```python
from build123d import *

# Parameters (mm, degrees)
SKETCH1_W           = 410
SKETCH1_H           = 70
BOSS_EXTRUDE1_DEPTH = 6
SKETCH2_W           = 6
SKETCH2_H           = 70
BOSS_EXTRUDE2_DEPTH = 25
SKETCH3_R           = 2.5
CUT_EXTRUDE1_DEPTH  = 418.891673384
SKETCH4_W           = 70
SKETCH4_H           = 8
CUT_EXTRUDE2_DEPTH  = 418.891673384


with BuildPart() as part:
    # Sketch1 → Boss-Extrude1 (new body)
    with BuildSketch(Plane(origin=(0, 0, 0), x_dir=(1, 0, 0), z_dir=(0, 1, 0))):
        with Locations((134.639039491, 39.648849176)):
            Rectangle(SKETCH1_W, SKETCH1_H)
    extrude(amount=BOSS_EXTRUDE1_DEPTH)

    # Sketch2 → Boss-Extrude2 (add)
    with BuildSketch(Plane(origin=(0, 6, 0), x_dir=(1, 0, 0), z_dir=(0, 1, 0))):
        with Locations((-67.360960509, 39.648849176)):
            Rectangle(SKETCH2_W, SKETCH2_H)
        with Locations((336.639039491, 39.648849176)):
            Rectangle(SKETCH2_W, SKETCH2_H)
    extrude(amount=BOSS_EXTRUDE2_DEPTH)

    # Sketch3 → Cut-Extrude1 (cut, through all)
    with BuildSketch(Plane.ZY.offset(70.360960509)):
        with Locations((-64.648849176, 16)):
            Circle(SKETCH3_R)
        with Locations((-14.648849176, 16)):
            Circle(SKETCH3_R)
    extrude(amount=-CUT_EXTRUDE1_DEPTH, mode=Mode.SUBTRACT)

    # Sketch4 → Cut-Extrude2 (cut, through all)
    with BuildSketch(Plane(origin=(339.639039491, 0, 0), x_dir=(0, 0, -1), z_dir=(1, 0, 0))):
        with Locations((39.648849176, 27)):
            Rectangle(SKETCH4_W, SKETCH4_H)
    extrude(amount=-CUT_EXTRUDE2_DEPTH, mode=Mode.SUBTRACT)


solid = part.part
```
Part model, mm, in its own coordinate system. A direction names the side the tool comes from. Round coordinates to 2 decimals unless told otherwise and drop trailing zeros. Loops run counter-clockwise (first coordinate to the right, second up) from the corner with the lowest first, then second, coordinate; pieces in that order, holes last.
Item 1: Cut at B-B, the plane z = -58.5. Give the cut face in (x, y).
Item 2: Cut at A-A, the plane y = 9.5. Give the cut face in (x, z).
Item 3: Drill centre lines: line 1 (X direction, y = 17.5, z = -54.5); line 2 (Y direction, x = 301.5, z = -68.5). Where is each one in solid material? Low to high.
Item 4: 3-axis set-ups, long thin cutter, end or side, ignore diameter. For faces 1 (the face through (333.639, 14, -39)), 2 (the face through (134, 2, -74.649)): which of +Z, -Z, +X, -X, +Y, -Y reach the whole face in a straight line?
Item 5: Cut at C-C, the plane x = 307. Give the cut face in (y, z).
Item 6: Mould opens along X. For faces 3 (the face through (-64.361, 14, -39)), 4 (the face through (339.639, 11, -39)), 5 (the face through (-70.361, 11, -39)), 6 (the face through (132, 0, -40)) say: +X half, -X half, draft (parallel to the pull), parting line (faces both ways), or undercut.
Item 7: Drop flat-ended pins along their axis: P1, Ø21, axis at x = 56.5, z = -52, coming from the +Y side; P2, Ø4.5, axis at y = 16, z = -14.65, coming from the +X side; P3, Ø6.5, axis at y = 16, z = -64.65, coming from the +X side. Give the stop position or say it passes through.
A:
1. outline: (-70.36, 0) - (339.64, 0) - (339.64, 23) - (333.64, 23) - (333.64, 6) - (-64.36, 6) - (-64.36, 23) - (-70.36, 23) - close
2. outline: (-70.36, -74.65) - (-64.36, -74.65) - (-64.36, -4.65) - (-70.36, -4.65) - close; (333.64, -74.65) - (339.64, -74.65) - (339.64, -4.65) - (333.64, -4.65) - close
3. line 1: x = -70.36 to -64.36, 333.64 to 339.64
3. line 2: y = 0 to 6
4. face 1: +Z, -Z, +Y
4. face 2: -Z, +X, -X, +Y, -Y
5. outline: (0, -74.65) - (6, -74.65) - (6, -4.65) - (0, -4.65) - close
6. face 3: undercut
6. face 4: +X half
6. face 5: -X half
6. face 6: draft
7. P1: stops at y = 6
7. P2: passes through
7. P3: stops at x = 339.64
